Geometry check sheet. Reference: drawing and pictorial views, mm from the part's lowest x, y, z. A direction names the side the tool comes from. Round coordinates to 2 decimals unless told otherwise and drop trailing zeros. Write each loop counter-clockwise with the first axis right and the second up, starting at its lowest first coordinate (ties: lowest second). Pieces come first, ordered by that corner, then holes. Notation, with made-up numbers: (56, 81.25) - (82, 81.25) arc R20 cw to (82, 94.25) - close; hole circle Ø4 at (60, -15.5). An arc over 180 degrees is marked (long way). Use one line per item in the form item = value. Start each with the question number.
1) Gauge pin test, flat ends, axial feed: P1, Ø2, axis at y = 9.525, z = 25.4, coming from the -X side; P2, Ø10, axis at x = 22, z = 15.5, coming from the +Y side (1 decimal); P3, Ø3, axis at y = 10, z = 20, coming from the +X side (1 decimal). Record the tip position at first contact, or that the pin passes through.
2) Scan lines: probe 1 along Y at (x, z) = (1.45, 25.4); probe 2 along X at (y, z) = (12, 23.5) (1 decimal). Record each from-to range of solid material in increasing order.
3) Section check B-B (z = 6.35). Record the boundary of the cut face in (x, y) (1 decimal), then the cut area to 3 significant figures.
4) Section check A-A (x = 7.75). Count the separate pieces of the cut face and the enclosed holes in it.
5) Set-up check for the marked faces 1 and 2: record each of +Z, -Z, +X, -X, +Y, -Y from which the full face is reachable in a straight line by a thin tool's end or side.
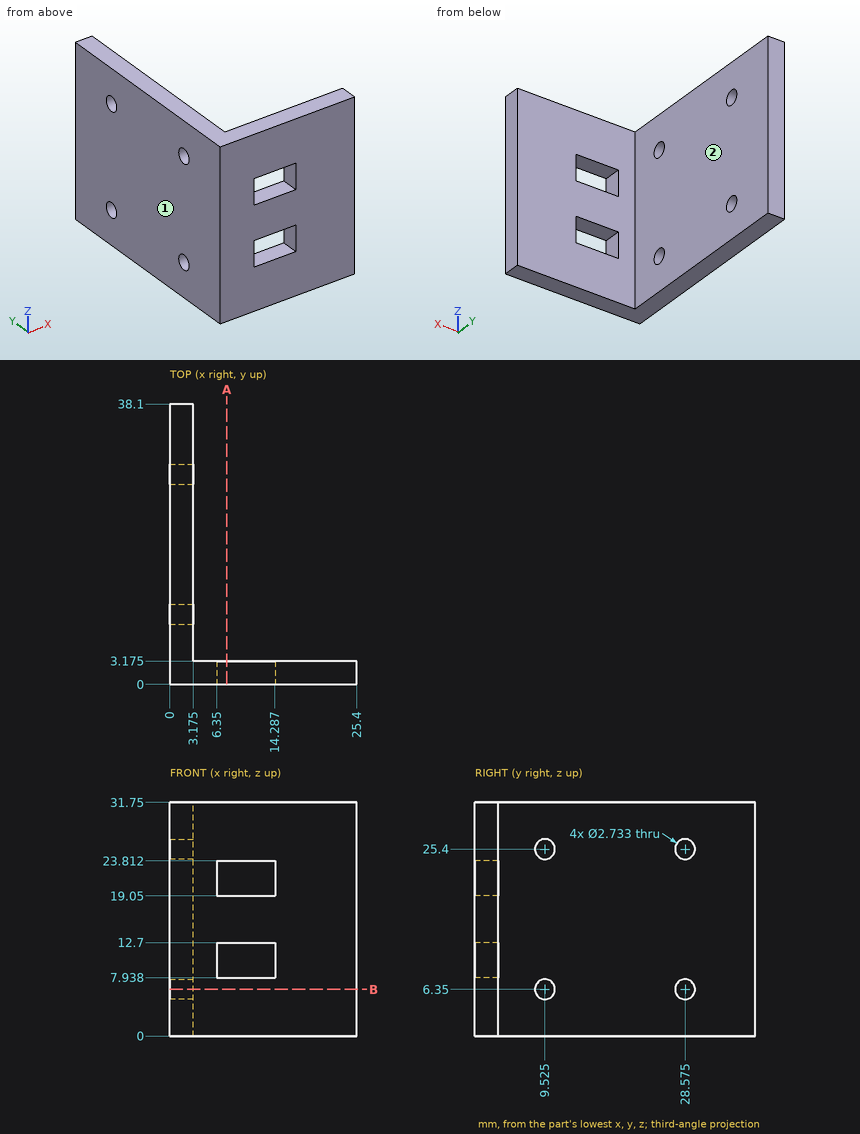
Results are:
q1.P1 = through
q1.P2 = 3.2
q1.P3 = 3.2
q2.probe_1 = 0 to 8.16, 10.89 to 27.21, 29.94 to 38.1
q2.probe_2 = 0 to 3.2
q3.outline = (0, 0) - (25.4, 0) - (25.4, 3.2) - (3.2, 3.2) - (3.2, 8.2) - (0, 8.2) - close; (0, 10.9) - (3.2, 10.9) - (3.2, 27.2) - (0, 27.2) - close; (0, 29.9) - (3.2, 29.9) - (3.2, 38.1) - (0, 38.1) - close
q3.area = 174 mm²
q4.separate_pieces = 3
q4.enclosed_holes = 0
q5.face_1 = +Z, -Z, -X, +Y, -Y
q5.face_2 = +Z, -Z, +X, +Y
